Work out the finished part from the listing and answer in its coordinate system (mm). A direction names the side the tool comes from. Give positions to 0.01 mm unless a question says otherwise; leave off trailing zeros. Write each loop counter-clockwise with the first axis right and the second up, starting at its lowest first coordinate (ties: lowest second). Pieces come first, ordered by that corner, then holes.
1) Straight lines are drawn through the part: probe 1 along Y at (x, z) = (0, 240) (3 decimals); probe 2 along X at (y, z) = (7.5, 319.5); probe 3 along Z at (x, y) = (164, 111.5). For each, find the intervals that lie inside material, in ascending order.
2) Given pin 1 Ø3 at (y, z) = (-50, 592.5) entering from +X; pin 2 Ø5 at (x, z) = (100, 342.5) entering from -Y; pin 3 Ø12 at (x, y) = (-48.5, -30.5) entering from -Z, each flat-ended and moving along its own axis, determine where each tip first touches the part or whether it passes through.
3) Find section B-B (x = 0). Determine the outline of the cut face in (y, z) (3 decimals), plus the area to 3 significant figures.
4) Determine the mould class of faces 1 (the face through (-159.127, 145.915, 504.019)), 2 (the face through (-3, 3, 1022.35)), 3 (the face through (-3, 3, 1016)) for opening direction Y: pulls with the +Y half, pulls with the -Y half, needs draft (parallel to the pull), parting line crosses it, or undercut.
5) A tool of negligible diameter and unlimited length cuts with its end or side. For faces 4 (the face through (-163.77, -125.58, 500.89)), 5 (the face through (111, -175, 0)), from which of +Z, -Z, +X, -X, +Y, -Y can it reach the whole face along a straight path? Write none if from no direction.
6) Find section A-A (z = 932.5). Determine the outline of the cut face in (x, y) (3 decimals).
```python
from build123d import *

# Parameters (mm, degrees)
F0_R     = 215.9
F0_R_2   = 206.375
F1_DEPTH = 457.2
F2_DEPTH = 1016
F3_R     = 215.9
F4_DEPTH = 6.35


with BuildPart() as f1:
    # F0 (on Top) → F1 (new body)
    with BuildSketch(Plane.XY):
        Circle(F0_R)
        Circle(F0_R_2, mode=Mode.SUBTRACT)
    extrude(amount=F1_DEPTH)

    # F0 (on Top) → F2 (join)
    with BuildSketch(Plane.XY):
        Circle(F0_R)
        Circle(F0_R_2, mode=Mode.SUBTRACT)
    extrude(amount=F2_DEPTH)

    # F3 (on face) → F4 (join)
    with BuildSketch(Plane.XY.offset(1016)):
        Circle(F3_R)
    extrude(amount=F4_DEPTH)


solid = f1.part
```
Results:
1. probe 1: y = -215.9 to -206.375, 206.375 to 215.9
1. probe 2: x = -215.77 to -206.24, 206.24 to 215.77
1. probe 3: z = 1016 to 1022.35
2. pin 1: stops at x = 210.38
2. pin 2: stops at y = -192.63
2. pin 3: stops at z = 1016
3. outline: (-215.9, 0) - (-206.375, 0) - (-206.375, 1016) - (206.375, 1016) - (206.375, 0) - (215.9, 0) - (215.9, 1022.35) - (-215.9, 1022.35) - close
3. area: 22,100 mm2
4. face 1: parting line crosses it
4. face 2: needs draft
4. face 3: undercut
5. face 4: -Z
5. face 5: -Z, +X, -X, +Y, -Y
6. outline: circle Ø431.8 at (0, 0); hole circle Ø412.75 at (0, 0)
